Could you check a few things on this model? Use its own coordinates, in mm. A direction names the side the tool comes from. Coordinates: 2 decimals unless noted, no trailing zeros. Loops run counter-clockwise (first coordinate to the right, second up) from the corner with the lowest first, then second, coordinate; pieces in that order, holes last. Notation, with made-up numbers: (24.25, 69.5) - (46.25, 69.5) arc R20 ccw to (46.25, 105.5) - close; hole circle Ø6 at (62, 21.25). An arc over 180 degrees is marked (long way). Use CSV: the item, a comma, the result in double quotes.
from build123d import *

# Parameters (mm, degrees)
SKETCH1_W           = 45
SKETCH1_H           = 65
SKETCH1_R           = 1.6
SKETCH1_W_2         = 3
SKETCH1_H_2         = 59
BOSS_EXTRUDE1_DEPTH = 2
CUT_EXTRUDE1_DEPTH  = 2.5


with BuildPart() as part:
    # Sketch1 → Boss-Extrude1 (new, symmetric)
    with BuildSketch(Plane(origin=(0, 0, 0), x_dir=(1, 0, 0), z_dir=(0, 1, 0))):
        Rectangle(SKETCH1_W, SKETCH1_H)
        with Locations(Location((-15, 27.5, 0), (0, 0, 270))):
            Circle(SKETCH1_R, mode=Mode.SUBTRACT)
        with Locations(Location((-15, 0, 0), (0, 0, 270))):
            Circle(SKETCH1_R, mode=Mode.SUBTRACT)
        with Locations(Location((-15, -27.5, 0), (0, 0, 90))):
            Circle(SKETCH1_R, mode=Mode.SUBTRACT)
        with Locations((-20, 0)):
            Rectangle(SKETCH1_W_2, SKETCH1_H_2, mode=Mode.SUBTRACT)
    extrude(amount=BOSS_EXTRUDE1_DEPTH, both=True)

    # Sketch4 → Cut-Extrude1 (cut)
    with BuildSketch(Plane.XZ.offset(2)):
        Polygon((-15, -3.319764048), (-12.125, -1.659882024), (-12.125, 1.659882024), (-15, 3.319764048), (-17.875, 1.659882024), (-17.875, -1.659882024), align=None)
        Polygon((-17.875, -25.840117976), (-15, -24.180235952), (-12.125, -25.840117976), (-12.125, -29.159882024), (-15, -30.819764048), (-17.875, -29.159882024), align=None)
        Polygon((-15, 24.180235952), (-12.125, 25.840117976), (-12.125, 29.159882024), (-15, 30.819764048), (-17.875, 29.159882024), (-17.875, 25.840117976), align=None)
    extrude(amount=-CUT_EXTRUDE1_DEPTH, mode=Mode.SUBTRACT)


solid = part.part
(1) Suppose I cut it at A-A (z = 27.5). Write out the boundary of the cut face in (x, y) (3 decimals).
Computed:
outline,"(-22.5, -2) - (-21.5, -2) - (-21.5, 2) - (-22.5, 2) - close; (-18.5, -2) - (-17.875, -2) - (-17.875, 0.5) - (-16.6, 0.5) - (-16.6, 2) - (-18.5, 2) - close; (-13.4, 0.5) - (-12.125, 0.5) - (-12.125, -2) - (22.5, -2) - (22.5, 2) - (-13.4, 2) - close"
(2) Which directions (+Z, -Z, +X, -X, +Y, -Y) give clear straight access to the entire face, cutting with the end or side of a thin tool? Please do faces 1 (the face through (-21.5, 0, 0)), 2 (the face through (-12.125, -1, -27)), 3 (the face through (5, 2, 0)).
Computed:
face 1,"+Y, -Y"
face 2,"-Y"
face 3,"+Z, -Z, +X, -X, +Y"
(3) Please list where these lines run through material, in increasing order: line 1 (X direction, y = 1.35, z = 0); line 2 (Z direction, x = -15, y = 1.05); line 3 (X direction, y = -1.1, z = -29) (3 decimals).
Computed:
line 1,"x = -22.5 to -21.5, -18.5 to -16.6, -13.4 to 22.5"
line 2,"z = -32.5 to -29.1, -25.9 to -1.6, 1.6 to 25.9, 29.1 to 32.5"
line 3,"x = -22.5 to -21.5, -18.5 to -17.875, -12.125 to 22.5"
(4) Thinking about a two-plate mould opening in Z: for faces 4 (the face through (0, 0, -32.5)), 5 (the face through (-12.125, -1, 27)), 6 (the face through (-13.58, -0.77, 25)), 7 (the face through (22.5, 0, 0)), which applies, +Z half, -Z half, draft (parallel to the pull), parting line (faces both ways), or undercut?
Computed:
face 4,"-Z half"
face 5,"undercut"
face 6,"undercut"
face 7,"draft"
(5) Will this pin go through, and if not, where does the flat tip stop? pin 1 (4 mm diameter, centred on x = -15, z = 0, fed in from -Y).
Computed:
pin 1,"stops at y = 0.5"
(6) Suppose I cut it at B-B (y = -1.2). Write out the boundary of the cut face in (x, z) (3 decimals), plus the area to 3 significant figures.
Computed:
outline,"(-22.5, -32.5) - (22.5, -32.5) - (22.5, 32.5) - (-22.5, 32.5) - close; hole (-21.5, -29.5) - (-18.5, -29.5) - (-18.5, 29.5) - (-21.5, 29.5) - close; hole (-17.875, -29.16) - (-15, -30.82) - (-12.125, -29.16) - (-12.125, -25.84) - (-15, -24.18) - (-17.875, -25.84) - close; hole (-17.875, -1.66) - (-15, -3.32) - (-12.125, -1.66) - (-12.125, 1.66) - (-15, 3.32) - (-17.875, 1.66) - close; hole (-17.875, 25.84) - (-15, 24.18) - (-12.125, 25.84) - (-12.125, 29.16) - (-15, 30.82) - (-17.875, 29.16) - close"
area,"2,660 mm²"
